For this review, take the finished solid that the model builds, in its own axes (mm). Face numbers are marked on the shaded views. Round coordinates to 2 decimals unless told otherwise and drop trailing zeros. Write each loop counter-clockwise with the first axis right and the second up, starting at its lowest first coordinate (ties: lowest second). Pieces come first, ordered by that corner, then holes. Notation, with made-up numbers: (86, 69.25) -> (125, 69.25) arc R16 cw to (125, 88.25) -> close; hole circle Ø2 at (16, -11.75). An arc over 180 degrees is marked (long way). Write each question's results on one line, items separated by ' | '. Start each with the question number.
Item 1: Add section B-B (z = 3.2). State the section outline as (x, y) points.
Item 2: Add section D-D (x = -3.5). State the section outline as (y, z) points.
Item 3: Add section A-A (y = 0). State the section outline as (x, z) points.
Item 4: Add section C-C (y = 12.5). State the section outline as (x, z) points, plus the area to 3 significant figures.
Item 5: To check wall thickness, follow line 1 along Y through (x, z) = (10, 2.5); line 2 along Y through (x, z) = (4.5, 2.1); line 3 along Y through (x, z) = (-18, 0.35). State the ranges of each line that lie inside material, in increasing order.
Item 6: Clearance check with a flat-ended pin moving along its axis: pin 1 (3 mm diameter, centred on y = 8.5, z = 4.5, fed in from -X). State where the tip first meets the part, or that it passes through.
Item 7: The part is to be moulded in two halves that separate along X. For the marked faces 1, 2 and 3, say which applies: +X half, -X half, draft (parallel to the pull), parting line (faces both ways), or undercut.
from build123d import *

# Parameters (mm, degrees)
SKETCH_1_R      = 1.5
EXTRUDE_1_DEPTH = 5.7


with BuildPart() as part:
    # 스케치1 → 보스-돌출1 (new body)
    with BuildSketch(Plane.XY):
        with BuildLine():
            Line((-5.980762114, 5), (10, 5))
            ThreePointArc((10, 5), (15, 0), (10, -5))
            Line((10, -5), (-10, -5))
            ThreePointArc((-10, -5), (-14.330127019, -2.5), (-14.330127019, 2.5))
            Line((-14.330127019, 2.5), (-26.400635095, 9.468911087))
            Line((-26.400635095, 9.468911087), (-30.308305875, 7.68355398))
            Line((-30.308305875, 7.68355398), (-33.400635095, 9.468911087))
            Line((-33.400635095, 9.468911087), (-36.492964314, 11.254268194))
            ThreePointArc((-36.492964314, 11.254268194), (-34.674569114, 16.481937097), (-29.150635095, 16.830127019))
            Line((-29.150635095, 16.830127019), (-10.980762114, 6.339745962))
            ThreePointArc((-10.980762114, 6.339745962), (-8.568952565, 5.340741737), (-5.980762114, 5))
        make_face()
        with Locations((-10, 0)):
            Circle(SKETCH_1_R, mode=Mode.SUBTRACT)
        with Locations((10, 0)):
            Circle(SKETCH_1_R, mode=Mode.SUBTRACT)
        with Locations((-31.650635095, 12.5)):
            Circle(SKETCH_1_R, mode=Mode.SUBTRACT)
    extrude(amount=EXTRUDE_1_DEPTH)


solid = part.part
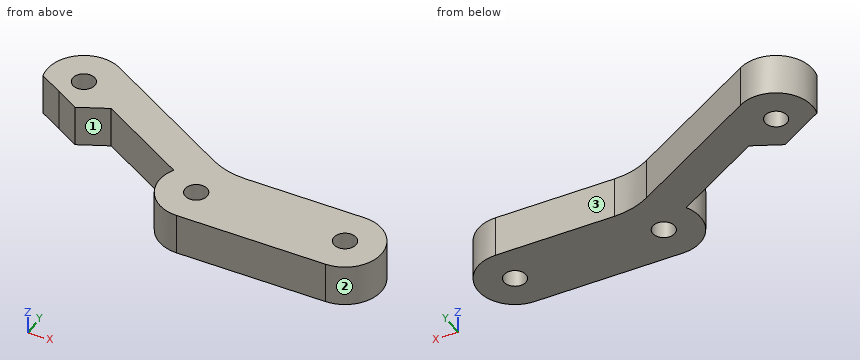
Responses:
1) outline: (-36.49, 11.25) -> (-30.31, 7.68) -> (-26.4, 9.47) -> (-14.33, 2.5) arc R5 ccw to (-10, -5) -> (10, -5) arc R5 ccw to (10, 5) -> (-5.98, 5) arc R10 cw to (-10.98, 6.34) -> (-29.15, 16.83) arc R5 ccw to start; hole circle Ø3 at (-31.65, 12.5); hole circle Ø3 at (-10, 0); hole circle Ø3 at (10, 0)
2) outline: (-5, 0) -> (5, 0) -> (5, 5.7) -> (-5, 5.7) -> close
3) outline: (-15, 0) -> (-11.5, 0) -> (-11.5, 5.7) -> (-15, 5.7) -> close; (-8.5, 0) -> (8.5, 0) -> (8.5, 5.7) -> (-8.5, 5.7) -> close; (11.5, 0) -> (15, 0) -> (15, 5.7) -> (11.5, 5.7) -> close
4) outline: (-36.65, 0) -> (-33.15, 0) -> (-33.15, 5.7) -> (-36.65, 5.7) -> close; (-30.15, 0) -> (-21.65, 0) -> (-21.65, 5.7) -> (-30.15, 5.7) -> close | area: 68.4 mm^2
5) line 1: y = -5 to -1.5, 1.5 to 5 | line 2: y = -5 to 5 | line 3: y = 4.62 to 10.39
6) pin 1: stops at x = -34.32
7) face 1: undercut | face 2: +X half | face 3: draft
